Geometry: final body of the model. Coordinates: model frame, mm. A direction names the side the tool comes from. Coordinates: 2 decimals unless noted, no trailing zeros. Loops run counter-clockwise (first coordinate to the right, second up) from the corner with the lowest first, then second, coordinate; pieces in that order, holes last. Notation, with made-up numbers: (44.25, 13.25) - (76.25, 13.25) arc R4 ccw to (76.25, 20.25) - close; hole circle Ø5 at (-9.5, -1). An arc over 180 degrees is marked (long way). Return JSON: item names as keys, results as strings.
Autodesk Fusion 360 part; units mm, degrees
sketch "Schizzo1" plane through (0, 0, 0) normal (0, 0, 1) x (1, 0, 0)
  line L0 (0, 0) -> (39.5, 0)
  line L1 (39.5, 0) -> (39.5, 36.4)
  line L2 (39.5, 36.4) -> (0, 36.4)
  line L3 (0, 36.4) -> (0, 0)
  dimension "d1" = 39.5
  dimension "d2" = 36.4
extrude "Estrusione1" add sketch "Schizzo1" along normal blind 4
sketch "Schizzo2" plane through (0, 0, 4) normal (0, 0, 1) x (-1, 0, 0)
  line L0 (0, -36.4) -> (0, 0)
  line L1 (0, 0) -> (-39.5, 0)
  line L2 (-39.5, 0) -> (-39.5, -36.4)
  line L3 (-39.5, -36.4) -> (0, -36.4)
  circle A0 centre (-19.75, -8.2) radius 2.55
  circle A1 centre (-19.75, -28.2) radius 2.55
  circle A2 centre (-19.75, -8.2) radius 4
  circle A3 centre (-19.75, -28.2) radius 4
  dimension "d5" = 5.1
  dimension "d6" = 5.1
  dimension "d7" = 8.2
  dimension "d8" = 19.75
  dimension "d9" = 8.2
  dimension "d10" = 19.75
  dimension "d11" = 8
  dimension "d12" = 8
extrude "Estrusione2" cut sketch "Schizzo2" against normal up to surface (4 mm away) contours A0
extrude "Estrusione3" cut sketch "Schizzo2" against normal up to surface (4 mm away) contours A1
extrude "Estrusione4" cut sketch "Schizzo2" against normal blind 2 contours A2 | A3
sketch "Schizzo3" plane through (0, 0, 4) normal (0, 0, 1) x (-1, 0, 0)
  circle A0 centre (-19.75, -8.2) radius 4
  circle A1 centre (-19.75, -28.2) radius 4
  line L0 (0, -36.4) -> (0, 0)
  line L1 (0, 0) -> (-39.5, 0)
  line L2 (-39.5, 0) -> (-39.5, -36.4)
  line L3 (-39.5, -36.4) -> (0, -36.4)
  line L4 (-39.5, -36.4) -> (0, -36.4)
  line L5 (0, -36.4) -> (0, -19.4)
  line L6 (0, -19.4) -> (-39.5, -19.4)
  line L7 (-39.5, -19.4) -> (-39.5, -36.4)
  circle A2 centre (-3, -23.4) radius 1.5
  circle A3 centre (-3, -33.4) radius 1.5
  circle A4 centre (-36.5, -33.4) radius 1.5
  circle A5 centre (-36.5, -33.4) radius 2.5
  circle A6 centre (-3, -33.4) radius 2.5
  circle A7 centre (-3, -23.4) radius 2.5
  dimension "d19" = 39.5
  dimension "d20" = 17
  dimension "d21" = 3
  dimension "d22" = 13
  dimension "d23" = 3
  dimension "d24" = 3
  dimension "d25" = 3
  dimension "d26" = 3
  dimension "d27" = 3
  dimension "d28" = 3
  dimension "d29" = 3
  dimension "d30" = 5
  dimension "d31" = 5
  dimension "d32" = 5
extrude "Estrusione5" add sketch "Schizzo3" along normal blind 4 contours A5 | A6 | A7
Item 1: First-contact query: pin 1 Ø1 at (x, z) = (34, 3.5) entering from -Y; pin 2 Ø9 at (x, y) = (19, 6.5) entering from +Z; pin 3 Ø6.5 at (x, y) = (19.75, 28.2) entering from +Z; pin 4 Ø1 at (x, z) = (34, 6.5) entering from +Y. Flat tips, straight axial feed; report the tip coordinate or a pass-through.
Worked out:
{"pin 1": "y = 0", "pin 2": "z = 4", "pin 3": "z = 2", "pin 4": "y = 34.9"}
Item 2: Mould query, pull axis X, two halves, no side actions, for faces 3 (the face through (17, 8, 2)), 4 (the face through (0, 18, 2)), 5 (the face through (20, 36.4, 2)), 6 (the face through (22.924, 10.634, 3.014)). Classes: +X half, -X half, draft (parallel to the pull), parting line (faces both ways), or undercut.
Worked out:
{"face 3": "undercut", "face 4": "-X half", "face 5": "draft", "face 6": "undercut"}
Item 3: Ray query, probe 1 along X at (y, z) = (33.4, 5.05); probe 2 along Y at (x, z) = (19.5, 2.75); probe 3 along Y at (x, z) = (3, 7). Return the intervals inside material, ascending. Write a range as from..to.
Worked out:
{"probe 1": "0.5..1.5, 4.5..5.5, 34..35, 38..39", "probe 2": "0..4.21, 12.19..24.21, 32.19..36.4", "probe 3": "20.9..21.9, 24.9..25.9, 30.9..31.9, 34.9..35.9"}
Item 4: Reachability of faces 1 (the face through (37.7, 32.5, 6)), 2 (the face through (1, 23, 8)) from +Z, -Z, +X, -X, +Y, -Y: full face, straight path, thin tool, end or side. Return the list, or none.
Worked out:
{"face 1": "+Z", "face 2": "+Z, +X, -X, +Y, -Y"}
Item 5: Section query B-B, the plane x = 19.75. Return loops of the section in (y, z), and give its area (3 significant figures).
Worked out:
{"outline": "(0, 0) - (5.65, 0) - (5.65, 2) - (4.2, 2) - (4.2, 4) - (0, 4) - close; (10.75, 0) - (25.65, 0) - (25.65, 2) - (24.2, 2) - (24.2, 4) - (12.2, 4) - (12.2, 2) - (10.75, 2) - close; (30.75, 0) - (36.4, 0) - (36.4, 4) - (32.2, 4) - (32.2, 2) - (30.75, 2) - close", "area": "93.2 mm^2"}
Item 6: Section query A-A, the plane z = 6.75. Return loops of the section in (x, y), and give its area (3 significant figures).
Worked out:
{"outline": "circle Ø5 at (3, 23.4); circle Ø5 at (3, 33.4); circle Ø5 at (36.5, 33.4); hole circle Ø3 at (3, 23.4); hole circle Ø3 at (3, 33.4); hole circle Ø3 at (36.5, 33.4)", "area": "37.7 mm^2"}
Item 7: Section query D-D, the plane y = 23.4. Return loops of the section in (x, z), and give its area (3 significant figures).
Worked out:
{"outline": "(0, 0) - (39.5, 0) - (39.5, 4) - (5.5, 4) - (5.5, 8) - (4.5, 8) - (4.5, 4) - (1.5, 4) - (1.5, 8) - (0.5, 8) - (0.5, 4) - (0, 4) - close", "area": "166 mm^2"}
Item 8: Section query C-C, the plane y = 10. Return loops of the section in (x, z), and give its area (3 significant figures).
Worked out:
{"outline": "(0, 0) - (17.94, 0) - (17.94, 2) - (16.18, 2) - (16.18, 4) - (0, 4) - close; (21.56, 0) - (39.5, 0) - (39.5, 4) - (23.32, 4) - (23.32, 2) - (21.56, 2) - close", "area": "136 mm^2"}
